Input: part model. Units: mm. Frame: model coordinates. A direction names the side the tool comes from. Give positions to 0.01 mm unless a question says otherwise; leave off trailing zeros. Write each loop counter-clockwise with the first axis right and the second up, starting at its lowest first coordinate (ties: lowest second). Pieces come first, ordered by that corner, then holes. Notation, with made-up numbers: (-16, 66) - (4, 66) arc R24 ccw to (4, 99) - close; hole circle Ø7 at (28.5, 45.25). An arc over 180 degrees is marked (long way). Answer as CSV lines item,"result". Start each with the question number.
from build123d import *

# Parameters (mm, degrees)
EXTRUDE1_DEPTH = 0.8
SKETCH2_W      = 4.6
SKETCH2_H      = 3
EXTRUDE2_DEPTH = 0.83


with BuildPart() as part:
    # Sketch1 → Extrude1 (new body)
    with BuildSketch(Plane.XY):
        with BuildLine():
            Line((1.197612835, -16.845933624), (4.197612835, -16.845933624))
            Line((4.197612835, -16.845933624), (4.197612835, -25.645933624))
            ThreePointArc((4.197612835, -25.645933624), (3.197612835, -26.645933624), (4.197612835, -27.645933624))
            Line((4.197612835, -27.645933624), (4.197612835, -36.445933624))
            Line((4.197612835, -36.445933624), (1.197612835, -36.445933624))
            ThreePointArc((1.197612835, -36.445933624), (0.197612835, -35.445933624), (-0.802387165, -36.445933624))
            Line((-0.802387165, -36.445933624), (-3.802387165, -36.445933624))
            Line((-3.802387165, -36.445933624), (-3.802387165, -27.645933624))
            ThreePointArc((-3.802387165, -27.645933624), (-2.802387165, -26.645933624), (-3.802387165, -25.645933624))
            Line((-3.802387165, -25.645933624), (-3.802387165, -16.845933624))
            Line((-3.802387165, -16.845933624), (-0.802387165, -16.845933624))
            ThreePointArc((-0.802387165, -16.845933624), (0.197612835, -17.845933624), (1.197612835, -16.845933624))
        make_face()
    extrude(amount=EXTRUDE1_DEPTH)

    # Sketch2 → Extrude2 (add)
    with BuildSketch(Plane.XY.offset(0.8)):
        with Locations((0.197612835, -20.645933624)):
            Rectangle(SKETCH2_W, SKETCH2_H)
        with Locations((0.197612835, -32.645933624)):
            Rectangle(SKETCH2_W, SKETCH2_H)
        with Locations((0.197612835, -24.645933624)):
            Rectangle(SKETCH2_W, SKETCH2_H)
        with Locations((0.197612835, -28.645933624)):
            Rectangle(SKETCH2_W, SKETCH2_H)
    extrude(amount=EXTRUDE2_DEPTH)


solid = part.part
1) Material intervals for line 1 (Y direction, x = 0.5, z = 1.05); line 2 (Z direction, x = 2, y = -18.25); line 3 (Y direction, x = 3.5, z = 0.45), sorted ascending. Write a range as from..to.
2) Pull-direction query (X, two-part tool) for faces 1 (the cylindrical face through (0.176, -17.846, 0.394)), 2 (the flat face through (2.498, -33, 1)), 3 (the flat face through (0, -25, 1.63)); classes: +X half, -X half, draft (parallel to the pull), parting line (faces both ways), or undercut.
3) Cut plane C-C on y = -33.75. Output: boundary loops of the cut face in (x, z).
4) Reachability of faces 4 (the flat face through (2.498, -25, 1)), 5 (the flat face through (0, -21, 1.63)), 6 (the cylindrical face through (3.2, -26.6, 0.4)), 7 (the flat face through (0, -31.146, 1)), 8 (the flat face through (-2.102, -29, 1)) from +Z, -Z, +X, -X, +Y, -Y: full face, straight path, thin tool, end or side. Return the list, or none.
5) Cut plane A-A on z = 1.3. Output: boundary loops of the cut face in (x, y), and give its area (3 significant figures).
6) Contact query for flat-ended pins moving along their axis: P1, Ø0.7, axis at y = -28, z = 1.5, coming from the +X side; P2, Ø0.9, axis at y = -24, z = 1.5, coming from the -X side; P3, Ø0.9, axis at y = -32, z = 1, coming from the -X side; P4, Ø0.7, axis at x = 1, z = 1.5, coming from the +Y side. Output: stop coordinate, or through.
7) Cut plane D-D on z = 0.25. Output: boundary loops of the cut face in (x, y).
8) Cut plane B-B on x = 3.5. Output: boundary loops of the cut face in (y, z).
Numbers:
1,line 1,"y = -34.15..-31.15, -30.15..-27.15, -26.15..-23.15, -22.15..-19.15"
1,line 2,"z = 0..0.8"
1,line 3,"y = -36.45..-27.36, -25.93..-16.85"
2,face 1,"undercut"
2,face 2,"+X half"
2,face 3,"draft"
3,outline,"(-3.8, 0) - (4.2, 0) - (4.2, 0.8) - (2.5, 0.8) - (2.5, 1.63) - (-2.1, 1.63) - (-2.1, 0.8) - (-3.8, 0.8) - close"
4,face 4,"+Z, +X, +Y, -Y"
4,face 5,"+Z, +X, -X, +Y, -Y"
4,face 6,"+Z, -Z, +X"
4,face 7,"+Z, +X, -X"
4,face 8,"+Z, -X, +Y, -Y"
5,outline,"(-2.1, -34.15) - (2.5, -34.15) - (2.5, -31.15) - (-2.1, -31.15) - close; (-2.1, -30.15) - (2.5, -30.15) - (2.5, -27.15) - (-2.1, -27.15) - close; (-2.1, -26.15) - (2.5, -26.15) - (2.5, -23.15) - (-2.1, -23.15) - close; (-2.1, -22.15) - (2.5, -22.15) - (2.5, -19.15) - (-2.1, -19.15) - close"
5,area,"55.2 mm²"
6,P1,"stops at x = 2.5"
6,P2,"stops at x = -2.1"
6,P3,"stops at x = -3.8"
6,P4,"stops at y = -19.15"
7,outline,"(-3.8, -36.45) - (-0.8, -36.45) arc R1 cw to (1.2, -36.45) - (4.2, -36.45) - (4.2, -27.65) arc R1 cw to (4.2, -25.65) - (4.2, -16.85) - (1.2, -16.85) arc R1 cw to (-0.8, -16.85) - (-3.8, -16.85) - (-3.8, -25.65) arc R1 cw to (-3.8, -27.65) - close"
8,outline,"(-36.45, 0) - (-27.36, 0) - (-27.36, 0.8) - (-36.45, 0.8) - close; (-25.93, 0) - (-16.85, 0) - (-16.85, 0.8) - (-25.93, 0.8) - close"
